Autodesk Inventor part; units mm, degrees
ref_plane "YZ Plane" through (0, 0, 0) normal (1, 0, 0) x (0, 1, 0)
ref_plane "XZ Plane" through (0, 0, 0) normal (0, 1, 0) x (-1, 0, 0)
ref_plane "XY Plane" through (0, 0, 0) normal (0, 0, 1) x (1, 0, 0)
sketch "Sketch1" plane through (0, 0, 0) normal (0, 0, 1) x (1, 0, 0)
  line L0 (0, 3.75) -> (2, 3.75)
  line L1 (2, 3.75) -> (2, -4)
  line L2 (2, -4) -> (0, -4)
  line L3 (0, -4) -> (0, 3.75) construction
  line L4 (0, -4) -> (-5, -4)
  line L5 (-5, -4) -> (-5, -1)
  line L6 (-5, -1) -> (0, -1)
  line L7 (0, 3.75) -> (-1, 3.75)
  line L8 (-1, 3.75) -> (-1, 0.75)
  line L9 (-1, 0.75) -> (0, 0.75)
  line L10 (0, 0.75) -> (0, 3.75) construction
  line L11 (0, 0.75) -> (0, -1)
  point P0 (0, 0)
  point P1 (0, -0.125)
  point P2 (1, 3.75)
  dimension "d0" = 4
  dimension "d1" = 2
  dimension "d5" = 5
  dimension "d6" = 1.75
  dimension "d7" = 3
  dimension "d11" = 3
  dimension "d12" = 3
extrude "Extrusion1" add sketch "Sketch1" along normal blind 243.25
sketch "Sketch2" plane through (-1, 0.75, 0) normal (-1, 0, 0) x (0, 0, 1)
  line L0 (0, 3) -> (0, 0)
  line L1 (0, 0) -> (243.25, 0)
  line L2 (243.25, 3) -> (243.25, 0)
  line L3 (0, 3) -> (243.25, 3)
  point P0 (0, -0.75)
extrude "Extrusion2" cut sketch "Sketch2" against normal blind 0.9
chamfer "Chamfer1" distance 2.5 angle 45 1 edges at (-5, -4, 121.625)
sketch "Sketch3" plane through (-0.1, 0.75, 0) normal (-1, 0, 0) x (0, 0, 1)
  line L0 (0, 3) -> (243.25, 3)
  line L1 (0, 3) -> (2.95, 3)
  line L2 (2.95, 3) -> (2.95, 1.05)
  line L3 (2.95, 1.05) -> (0, 1.05)
  line L4 (0, 1.05) -> (0, 3)
  line L5 (59.8466, 2.85) -> (59.8466, 0.85) construction
  line L6 (59.8466, 2.85) -> (59.8466, 3) construction
  line L7 (59.8466, 3) -> (64.7966, 3)
  line L8 (64.7966, 3) -> (64.7966, 1.05)
  line L9 (64.7966, 1.05) -> (59.8466, 1.05)
  line L10 (59.8466, 1.05) -> (59.8466, 3)
  line L11 (243.25, 3) -> (243.25, 0)
  line L12 (243.25, 3) -> (240.3, 3)
  line L13 (240.3, 3) -> (240.3, 1.05)
  line L14 (240.3, 1.05) -> (243.25, 1.05)
  line L15 (243.25, 1.05) -> (243.25, 3)
  point P0 (0, -0.75)
  point P1 (243.25, 1.05)
  dimension "d18" = 1.95
  dimension "d19" = 2.95
  dimension "d20" = 4.95
  dimension "d21" = 1.95
  dimension "d22" = 1.95
  dimension "d23" = 2.95
extrude "Extrusion3" add sketch "Sketch3" along normal blind 2.95
sketch "Sketch4" plane through (2, -4, 0) normal (0, -1, 0) x (1, 0, 0)
  circle A0 centre (-4.4525, -10.6025) radius 0.725 construction
  line L0 (-3.2, -15.005) -> (-3.2, -1) construction
  line L1 (-4.5, 0) -> (0, 0) construction
  line L2 (-4.5, 243.25) -> (0, 243.25) construction
  circle A1 centre (-10.2025, 230.7475) radius 2.55 construction
  circle A2 centre (-10.1275, 141.3958) radius 2.55 construction
  circle A3 centre (-10.2025, 51.9975) radius 2.55 construction
  circle A4 centre (-10.2025, 29.9975) radius 2.55 construction
  circle A5 centre (-10.2025, 10.9975) radius 2.55 construction
  line L3 (-3.2, 6.8975) -> (-7, 6.8975)
  line L4 (-7, 6.8975) -> (-7, 16.8975)
  line L5 (-7, 16.8975) -> (-3.2, 16.8975)
  line L6 (-3.2, 16.8975) -> (-3.2, 6.8975)
  line L7 (-3.2, 25.8975) -> (-7, 25.8975)
  line L8 (-7, 25.8975) -> (-7, 35.8975)
  line L9 (-7, 35.8975) -> (-3.2, 35.8975)
  line L10 (-3.2, 35.8975) -> (-3.2, 25.8975)
  line L11 (-3.2, 47.8975) -> (-7, 47.8975)
  line L12 (-7, 47.8975) -> (-7, 57.8975)
  line L13 (-7, 57.8975) -> (-3.2, 57.8975)
  line L14 (-3.2, 57.8975) -> (-3.2, 47.8975)
  line L15 (-3.2, 137.2957) -> (-7, 137.2957)
  line L16 (-7, 137.2957) -> (-7, 147.2957)
  line L17 (-7, 147.2957) -> (-3.2, 147.2957)
  line L18 (-3.2, 147.2957) -> (-3.2, 137.2957)
  line L19 (-2.1, 243.25) -> (-2.1, 0)
  line L20 (-2.1, 236.6475) -> (-2.1, 226.6475)
  circle A6 centre (-10.2025, -8.0025) radius 2.55 construction
  circle A7 centre (-5.5025, -3.6025) radius 0.725 construction
  line L21 (-3.2, -12.1025) -> (-10.2025, -12.1025) construction
  line L22 (-10.2025, -12.1025) -> (-10.2025, -2.1025) construction
  line L23 (-10.2025, -2.1025) -> (-3.2, -2.1025) construction
  line L24 (-7, 243.25) -> (-7, 0) construction
  line L25 (-7, 0) -> (-7, 243.25)
  line L26 (-7, 226.6475) -> (-3.2, 226.6475)
  line L27 (-3.2, 226.6475) -> (-3.2, 236.6475)
  line L28 (-3.2, 236.6475) -> (-7, 236.6475)
  line L29 (-7, 236.6475) -> (-7, 226.6475)
  point P0 (-2, 0)
  dimension "d26" = 1.5
  dimension "d27" = 1.5
  dimension "d28" = 4.1
  dimension "d29" = 5.9
  dimension "d30" = 4.1
  dimension "d31" = 5.9
  dimension "d32" = 4.1
  dimension "d33" = 5.9
  dimension "d34" = 4.1
  dimension "d35" = 5.9
  dimension "d36" = 4.1
  dimension "d37" = 5.9
  dimension "d40" = 4.1
  dimension "d41" = 5.9
extrude "Extrusion4" cut sketch "Sketch4" against normal up to surface (3 mm away)
equation "\"d30\" = d28"
equation "\"d31\" = d29"
equation "\"d32\" = d28"
equation "\"d33\" = d29"
equation "\"d34\" = d28"
equation "\"d35\" = d29"
equation "\"d36\" = d28"
equation "\"d37\" = d29"
equation "\"d40\" = d28"
equation "\"d41\" = d29"
properties part number "Case Rail" material "PET Plastic"
Verification items for the finished model (mm, model axes). Round coordinates to 2 decimals unless told otherwise and drop trailing zeros. Write each loop counter-clockwise with the first axis right and the second up, starting at its lowest first coordinate (ties: lowest second). Pieces come first, ordered by that corner, then holes. Notation, with made-up numbers: (42, 75) -> (71, 75) arc R21 cw to (71, 102) -> close; hole circle Ø10 at (-7.5, 26.5). An arc over 180 degrees is marked (long way). Write each question's results on one line, items separated by ' | '.
Q1. Sectioned sample at A-A, the plane z = 114.5. Record the boundary of the cut face in (x, y).
Derived:
outline: (-5, -1.5) -> (-2.5, -4) -> (2, -4) -> (2, 3.75) -> (-0.1, 3.75) -> (-0.1, 0.75) -> (0, 0.75) -> (0, -1) -> (-5, -1) -> close
Q2. Sectioned sample at B-B, the plane z = 142. Record the boundary of the cut face in (x, y).
Derived:
outline: (-1.2, -4) -> (2, -4) -> (2, 3.75) -> (-0.1, 3.75) -> (-0.1, 0.75) -> (0, 0.75) -> (0, -1) -> (-1.2, -1) -> close
Q3. Thickness scan on probe 1 along Z at (x, y) = (-0.75, 2); probe 2 along Z at (x, y) = (-3.5, -1.5); probe 3 along X at (y, z) = (-0.5, 132). Record the ranges inside material, lowest first.
Derived:
probe 1: z = 0 to 2.95, 59.85 to 64.8, 240.3 to 243.25 | probe 2: z = 0 to 6.9, 16.9 to 25.9, 35.9 to 47.9, 57.9 to 137.3, 147.3 to 226.65, 236.65 to 243.25 | probe 3: x = 0 to 2
Q4. Go/stop test with a flat-tipped pin: pin 1 Ø3.5 at (y, z) = (-2, 144.5) entering from -X. Record where the tip stops, or that it passes through.
Derived:
pin 1: stops at x = -1.2
